Can you work these out from the model? Positions are in its coordinate system, mm. Face numbers are marked on the shaded views. A direction names the side the tool comes from. Coordinates: 2 decimals unless noted, no trailing zeros. Order: outer loops, then holes, each group sorted by start corner. A loop starts at its lowest first (then second) coordinate and runs counter-clockwise, first axis right, second up. Notation, with made-up numbers: (11, -14) -> (61, -14) arc R8 cw to (61, -3) -> close; hole circle Ø3 at (7, 37.25). An arc over 180 degrees is marked (long way). Answer as CSV lines item,"result".
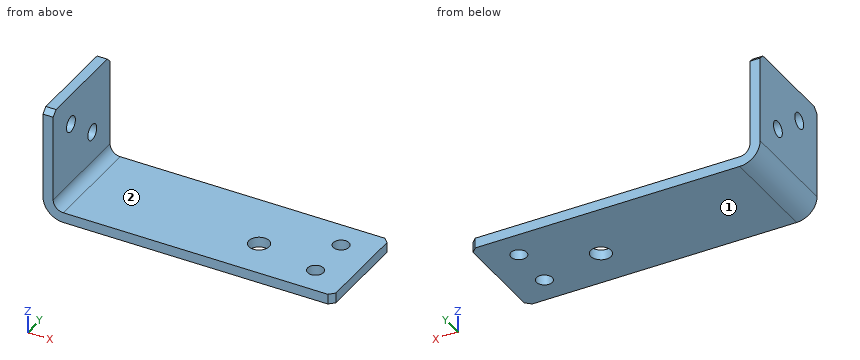
from build123d import *

# Parameters (mm, degrees)
BASE_DEPTH           = 20
SKETCH2_R            = 1.55
GUIDESIDEHOLES_DEPTH = 20
SKETCH3_R            = 1.55
FOOTSIDEHOLES_DEPTH  = 63.521996129
CHAMFER1_SIZE        = 1
SKETCH4_R            = 2
CABLETIEHOLE_DEPTH   = 63.521996129


with BuildPart() as part:
    # Sketch1 → Base (new body)
    with BuildSketch(Plane(origin=(0, 0, 0), x_dir=(1, 0, 0), z_dir=(0, 1, 0))):
        with BuildLine():
            Line((0, 0), (0, 18))
            ThreePointArc((0, 18), (0.585786438, 19.414213562), (2, 20))
            Line((2, 20), (55, 20))
            Line((55, 20), (55, 22))
            Line((55, 22), (2, 22))
            ThreePointArc((2, 22), (-0.828427125, 20.828427125), (-2, 18))
            Line((-2, 18), (-2, 0))
            Line((-2, 0), (0, 0))
        make_face()
    extrude(amount=BASE_DEPTH)

    # Sketch2 → GuideSideHoles (cut)
    with BuildSketch(Plane.ZY.offset(2)):
        with Locations((-12, 13.75)):
            Circle(SKETCH2_R)
        with Locations((-6, 6.25)):
            Circle(SKETCH2_R)
    extrude(amount=-GUIDESIDEHOLES_DEPTH, mode=Mode.SUBTRACT)

    # Sketch3 → FootSideHoles (cut, through all)
    with BuildSketch(Plane(origin=(0, 0, -22), x_dir=(-1, 0, 0), z_dir=(0, 0, -1))):
        with Locations((-48.5, 14.5)):
            Circle(SKETCH3_R)
        with Locations((-48.5, 5.5)):
            Circle(SKETCH3_R)
    extrude(amount=-FOOTSIDEHOLES_DEPTH, mode=Mode.SUBTRACT)

    # Chamfer1
    chamfer1_edges = [part.edges().sort_by_distance(p)[0] for p in [
        (-1, 0, 0),
        (55, 0, -21),
        (-1, 20, 0),
        (55, 20, -21),
    ]]
    chamfer(chamfer1_edges, length=CHAMFER1_SIZE)

    # Sketch4 → CableTieHole (cut, through all)
    with BuildSketch(Plane(origin=(0, 0, -22), x_dir=(-1, 0, 0), z_dir=(0, 0, -1))):
        with Locations((-36, 8)):
            Circle(SKETCH4_R)
    extrude(amount=-CABLETIEHOLE_DEPTH, mode=Mode.SUBTRACT)


solid = part.part
Q1. Imagine slicing it at C-C (z = -6). List the corners of the cut face in (x, y) for me, and give its area (3 significant figures).
Solution:
outline,"(-2, 0) -> (0, 0) -> (0, 4.7) -> (-2, 4.7) -> close; (-2, 7.8) -> (0, 7.8) -> (0, 20) -> (-2, 20) -> close"
area,"33.8 mm2"
Q2. Imagine slicing it at A-A (x = 36). List the corners of the cut face in (y, z) for me.
Solution:
outline,"(0, -22) -> (6, -22) -> (6, -20) -> (0, -20) -> close; (10, -22) -> (20, -22) -> (20, -20) -> (10, -20) -> close"
Q3. Imagine slicing it at B-B (x = 48.5). List the corners of the cut face in (y, z) for me.
Solution:
outline,"(0, -22) -> (3.95, -22) -> (3.95, -20) -> (0, -20) -> close; (7.05, -22) -> (12.95, -22) -> (12.95, -20) -> (7.05, -20) -> close; (16.05, -22) -> (20, -22) -> (20, -20) -> (16.05, -20) -> close"
Q4. If I drill on line 1 (Y direction, x = 48.5, z = -21.5); line 2 (X direction, y = 2.25, z = -6.75); line 3 (Y direction, x = 36, z = -20.75), over which ranges is the centre line in solid material (lowest first)?
Solution:
line 1,"0 to 3.95, 7.05 to 12.95, 16.05 to 20"
line 2,"-2 to 0"
line 3,"0 to 6, 10 to 20"
Q5. For P1, Ø2.5, axis at x = 48.5, y = 5.5, coming from the +Z side; P2, Ø6.5, axis at x = 36, y = 8, coming from the +Z side; P3, Ø3, axis at y = 12.5, z = -10.5, coming from the +X side, each with a flat end and sliding along its axis, tell me the tip position at first contact or that it passes through.
Solution:
P1,"through"
P2,"z = -20"
P3,"x = 0"
Q6. Which directions (+Z, -Z, +X, -X, +Y, -Y) give clear straight access to the entire face, cutting with the end or side of a thin tool? Please do the marked faces 1 and 2.
Solution:
face 1,"-Z, +X, -X, +Y, -Y"
face 2,"+Z, +X, +Y, -Y"
Q7. Imagine slicing it at D-D (y = 14.5). List the corners of the cut face in (x, z) for me.
Solution:
outline,"(-2, -18) arc R4 ccw to (2, -22) -> (46.95, -22) -> (46.95, -20) -> (2, -20) arc R2 cw to (0, -18) -> (0, -13.36) -> (-2, -13.36) -> close; (-2, -10.64) -> (0, -10.64) -> (0, 0) -> (-2, 0) -> close; (50.05, -22) -> (55, -22) -> (55, -20) -> (50.05, -20) -> close"
